Could you check a few things on this model? Use its own coordinates, in mm. A direction names the side the tool comes from. Coordinates: 2 decimals unless noted, no trailing zeros. Loops run counter-clockwise (first coordinate to the right, second up) from the corner with the lowest first, then second, coordinate; pieces in that order, holes last. Notation, with made-up numbers: (40, 65.25) - (54, 65.25) arc R18 ccw to (54, 69.25) - close; hole circle Ø8 at (13, 60.5). An arc over 180 degrees is marked (long way). One line per item, written item: value. Start each with the question number.
(1) If we mould it in two halves opening along X, with no side actions, what happens to faces 1 (the face through (-2.9, 47, 14)), 2 (the face through (0, 39, 13)), 3 (the face through (-2, 12, 15.5))? For each: pulls with the +X half, pulls with the -X half, needs draft (parallel to the pull), parting line crosses it, or undercut.
(2) If I drill on line 1 along Y through (x, z) = (-2.85, 7); line 2 along Y through (x, z) = (-0.3, 7); line 3 along Z through (x, y) = (-2.4, 23), over which ranges is the centre line in solid material (lowest first)? Write a range as from..to.
(3) I'm going to push flat-ended pins straight in: P1, Ø8, axis at y = 29, z = 6.5, coming from the -X side; P2, Ø1.2, axis at x = -3, y = 11, coming from the +Z side; P3, Ø2, axis at x = -2.5, z = 20, coming from the -Y side. Where does each tip first touch, or does it pass through?
(4) If we section it at D-D on x = -2.05: Write out the boundary of the cut face in (y, z).
(5) If we section it at C-C on z = 7.75: Write out the boundary of the cut face in (x, y), then the cut area to 3 significant figures.
(6) If we section it at A-A on y = 29.5: Write out the boundary of the cut face in (x, z).
(7) On a 3-axis mill with a long thin cutter (end or side, diameter ignored), from which of +Z, -Z, +X, -X, +Y, -Y can I reach the whole of each face in a straight line? I mean faces 4 (the face through (-2, 24, 21)), 5 (the face through (-2, 63, 13)), 6 (the face through (-1.4, 26, 5)). Say none if no direction works.
(8) If we section it at B-B on z = 16.5: Write out the boundary of the cut face in (x, y).
```python
from build123d import *

# Parameters (mm, degrees)
SKETCH1_W                                        = 30
SKETCH1_H                                        = 63
BOSS_EXTRUDE1_DEPTH                              = 3.9
SKETCH2_R                                        = 5
CUT_EXTRUDE1_DEPTH                               = 70.887123277
F_4_0_4_DIAMETER_HOLE1_D                         = 4
SKETCH12_W                                       = 14.5
SKETCH12_H                                       = 24
CUT_EXTRUDE2_DEPTH                               = 70.887123277
CBORE_FOR_M3_PAN_HEAD_MACHINE_SCREW2_D           = 3.2
CBORE_FOR_M3_PAN_HEAD_MACHINE_SCREW2_CBORE_D     = 9
CBORE_FOR_M3_PAN_HEAD_MACHINE_SCREW2_CBORE_DEPTH = 1
CSK_FOR_M3_FLAT_HEAD_MACHINE_SCREW1_D            = 3.2
CSK_FOR_M3_FLAT_HEAD_MACHINE_SCREW1_CSINK_D      = 4
CSK_FOR_M3_FLAT_HEAD_MACHINE_SCREW1_CSINK_ANGLE  = 90
SKETCH19_W                                       = 4
SKETCH19_H                                       = 39
CUT_EXTRUDE3_DEPTH                               = 70.887123277
SKETCH20_R                                       = 5
SKETCH20_R_2                                     = 3.5
BOSS_EXTRUDE2_DEPTH                              = 1.4


with BuildPart() as part:
    # Sketch1 → Boss-Extrude1 (new body)
    with BuildSketch(Plane(origin=(0, 0, 0), x_dir=(0, 0, -1), z_dir=(1, 0, 0))):
        with Locations((-15, 31.5)):
            Rectangle(SKETCH1_W, SKETCH1_H)
    extrude(amount=-BOSS_EXTRUDE1_DEPTH)

    # Sketch2 → Cut-Extrude1 (cut, through all)
    with BuildSketch(Plane(origin=(0, 0, 0), x_dir=(0, 0, -1), z_dir=(1, 0, 0))):
        with Locations((-7, 29.5)):
            Circle(SKETCH2_R)
    extrude(amount=-CUT_EXTRUDE1_DEPTH, mode=Mode.SUBTRACT)

    # Ø4.0 (4) Diameter Hole1 (through all)
    with Locations(Plane(origin=(0, 4.5, 7), x_dir=(0, 0, 1), z_dir=(1, 0, 0))):
        with Locations((0, 0)):
            Hole(F_4_0_4_DIAMETER_HOLE1_D / 2)

    # Sketch12 → Cut-Extrude2 (cut, through all)
    with BuildSketch(Plane(origin=(0, 0, 0), x_dir=(0, 0, -1), z_dir=(1, 0, 0))):
        with Locations((-22.75, 12)):
            Rectangle(SKETCH12_W, SKETCH12_H)
    extrude(amount=-CUT_EXTRUDE2_DEPTH, mode=Mode.SUBTRACT)

    # CBORE for M3 Pan Head Machine Screw2 (through all)
    with Locations(Plane(origin=(-3.9, 47.360571099, 16), x_dir=(0, 0, -1), z_dir=(-1, 0, 0))):
        with Locations((0, 0)):
            CounterBoreHole(CBORE_FOR_M3_PAN_HEAD_MACHINE_SCREW2_D / 2, CBORE_FOR_M3_PAN_HEAD_MACHINE_SCREW2_CBORE_D / 2, CBORE_FOR_M3_PAN_HEAD_MACHINE_SCREW2_CBORE_DEPTH)

    # CSK for M3 Flat Head Machine Screw1 (through all)
    with Locations(Plane(origin=(0, 36.032608687, 19.33966579), x_dir=(0, 0, 1), z_dir=(1, 0, 0))):
        with Locations((0, 0), (-14.431341448, -7.272)):
            CounterSinkHole(CSK_FOR_M3_FLAT_HEAD_MACHINE_SCREW1_D / 2, CSK_FOR_M3_FLAT_HEAD_MACHINE_SCREW1_CSINK_D / 2, counter_sink_angle=CSK_FOR_M3_FLAT_HEAD_MACHINE_SCREW1_CSINK_ANGLE)

    # Sketch19 → Cut-Extrude3 (cut, through all)
    with BuildSketch(Plane.ZY.offset(3.9)):
        with Locations((28, 43.5)):
            Rectangle(SKETCH19_W, SKETCH19_H)
    extrude(amount=-CUT_EXTRUDE3_DEPTH, mode=Mode.SUBTRACT)

    # Sketch20 → Boss-Extrude2 (add)
    with BuildSketch(Plane(origin=(0, 0, 0), x_dir=(0, 0, -1), z_dir=(1, 0, 0))):
        with Locations((-7, 29.5)):
            Circle(SKETCH20_R)
        with Locations((-7, 29.5)):
            Circle(SKETCH20_R_2, mode=Mode.SUBTRACT)
    extrude(amount=-BOSS_EXTRUDE2_DEPTH)


solid = part.part
```
Values:
1. face 1: pulls with the -X half
1. face 2: pulls with the +X half
1. face 3: needs draft
2. line 1: y = 0..2.5, 6.5..24.5, 34.5..63
2. line 2: y = 0..2.5, 6.5..26, 33..63
2. line 3: z = 0..15.5
3. P1: stops at x = -1.4
3. P2: stops at z = 15.5
3. P3: stops at y = 24
4. outline: (0, 0) - (63, 0) - (63, 26) - (24, 26) - (24, 15.5) - (0, 15.5) - close; hole circle Ø4 at (4.5, 7); hole circle Ø10 at (29.5, 7); hole circle Ø3.2 at (36.03, 19.34); hole circle Ø3.2 at (43.3, 4.91); hole circle Ø3.2 at (47.36, 16)
5. outline: (-3.9, 0) - (0, 0) - (0, 2.65) - (-3.9, 2.65) - close; (-3.9, 6.35) - (0, 6.35) - (0, 26.08) - (-1.4, 26.08) - (-1.4, 24.56) - (-3.9, 24.56) - close; (-3.9, 34.44) - (-1.4, 34.44) - (-1.4, 32.92) - (0, 32.92) - (0, 63) - (-3.9, 63) - close
5. area: 197 mm2
6. outline: (-3.9, 0) - (0, 0) - (0, 3.5) - (-1.4, 3.5) - (-1.4, 2) - (-3.9, 2) - close; (-3.9, 12) - (-1.4, 12) - (-1.4, 10.5) - (0, 10.5) - (0, 26) - (-3.9, 26) - close
7. face 4: +Z, +X, -X, -Y
7. face 5: +Z, -Z, +X, -X, +Y
7. face 6: -X
8. outline: (-3.9, 24) - (0, 24) - (0, 45.84) - (-2.9, 45.84) - (-2.9, 42.89) - (-3.9, 42.89) - close; (-3.9, 51.83) - (-2.9, 51.83) - (-2.9, 48.88) - (0, 48.88) - (0, 63) - (-3.9, 63) - close
